Could you check a few things on this model? Use its own coordinates, in mm. Round coordinates to 2 decimals unless told otherwise and drop trailing zeros. Loops run counter-clockwise (first coordinate to the right, second up) from the corner with the lowest first, then second, coordinate; pieces in that order, holes last.
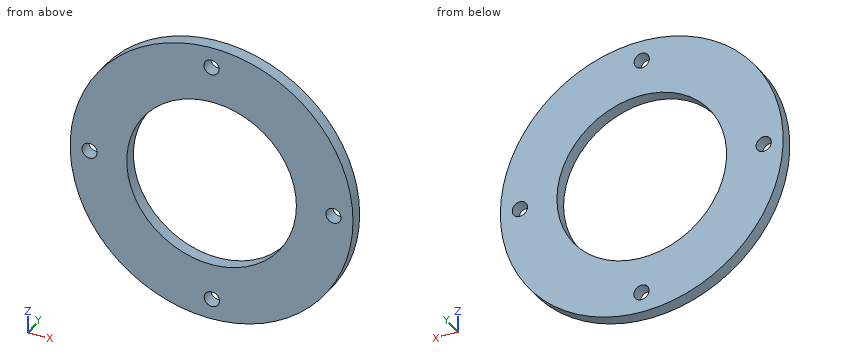
from build123d import *

# Parameters (mm, degrees)
SKETCH1_R                = 32.5
SKETCH1_R_2              = 19.5
BOSS_EXTRUDE2_DEPTH      = 3
SKETCH2_R                = 1.75
CUT_EXTRUDE2_DEPTH       = 1
CUT_EXTRUDE2_DEPTH_BACK  = 4
SKETCH5_R                = 1.75
CUT_EXTRUDE4_DEPTH       = 1
CUT_EXTRUDE4_DEPTH_BACK  = 4
SKETCH13_R               = 1.75
CUT_EXTRUDE12_DEPTH      = 1
CUT_EXTRUDE12_DEPTH_BACK = 4


with BuildPart() as part:
    # Sketch1 → Boss-Extrude2 (new body)
    with BuildSketch(Plane(origin=(0, 0, 0), x_dir=(1, 0, 0), z_dir=(0, 1, 0))):
        Circle(SKETCH1_R)
        Circle(SKETCH1_R_2, mode=Mode.SUBTRACT)
    extrude(amount=BOSS_EXTRUDE2_DEPTH)

    # Sketch2 → Cut-Extrude2 (cut, two sides)
    with BuildSketch(Plane(origin=(0, 3, 0), x_dir=(1, 0, 0), z_dir=(0, 1, 0))) as cut_extrude2_sk:
        with Locations((0, -27.788884535)):
            Circle(SKETCH2_R)
    extrude(amount=CUT_EXTRUDE2_DEPTH, mode=Mode.SUBTRACT)
    extrude(cut_extrude2_sk.sketch, amount=-CUT_EXTRUDE2_DEPTH_BACK, mode=Mode.SUBTRACT)

    # Sketch5 → Cut-Extrude4 (cut, two sides)
    with BuildSketch(Plane(origin=(0, 3, 0), x_dir=(1, 0, 0), z_dir=(0, 1, 0))) as cut_extrude4_sk:
        with Locations((0.057759675, 27.766269398)):
            Circle(SKETCH5_R)
    extrude(amount=CUT_EXTRUDE4_DEPTH, mode=Mode.SUBTRACT)
    extrude(cut_extrude4_sk.sketch, amount=-CUT_EXTRUDE4_DEPTH_BACK, mode=Mode.SUBTRACT)

    # Sketch13 → Cut-Extrude12 (cut, two sides)
    with BuildSketch(Plane(origin=(0, 3, 0), x_dir=(1, 0, 0), z_dir=(0, 1, 0))) as cut_extrude12_sk:
        with Locations((-28.027387252, -0.003979104)):
            Circle(SKETCH13_R)
        with Locations((28.01619309, 0)):
            Circle(SKETCH13_R)
    extrude(amount=CUT_EXTRUDE12_DEPTH, mode=Mode.SUBTRACT)
    extrude(cut_extrude12_sk.sketch, amount=-CUT_EXTRUDE12_DEPTH_BACK, mode=Mode.SUBTRACT)


solid = part.part
Item 1: Will these pins go through, and if not, where does the flat tip stop? pin 1 (12 mm diameter, centred on x = 1, z = 25, fed in from -Y); pin 2 (1.5 mm diameter, centred on y = 1, z = -19.5, fed in from -X); pin 3 (1 mm diameter, centred on x = -11.5, y = 1, fed in from -Z); pin 4 (1 mm diameter, centred on x = 7, y = 1, fed in from -Z).
Results list:
pin 1: stops at y = 0
pin 2: stops at x = -26.55
pin 3: stops at z = -30.58
pin 4: stops at z = -31.84
Item 2: If we section it at A-A, the plane x = -2.5: Please give me the cut outline in (y, z).
Results list:
outline: (0, -32.4) - (3, -32.4) - (3, -19.34) - (0, -19.34) - close; (0, 19.34) - (3, 19.34) - (3, 32.4) - (0, 32.4) - close
Item 3: If we section it at D-D, the plane z = -21.5: Please give me the cut outline in (x, y), then the cut area to 3 significant figures.
Results list:
outline: (-24.37, 0) - (24.37, 0) - (24.37, 3) - (-24.37, 3) - close
area: 146 mm2
Item 4: If I drill on line 1 along Z through (x, y) = (0, 0.6); line 2 along X through (y, z) = (1.45, 0); line 3 along Z through (x, y) = (0.5, 0.75), over which ranges is the centre line in solid material (lowest first)?
Results list:
line 1: z = -32.5 to -29.52, -26.02 to -19.5, 19.5 to 26.04, 29.54 to 32.5
line 2: x = -32.5 to -29.78, -26.28 to -19.5, 19.5 to 26.27, 29.77 to 32.5
line 3: z = -32.5 to -29.46, -26.07 to -19.49, 19.49 to 26.11, 29.47 to 32.5
Item 5: If we section it at B-B, the plane z = -5.5: Please give me the cut outline in (x, y), then the cut area to 3 significant figures.
Results list:
outline: (-32.03, 0) - (-18.71, 0) - (-18.71, 3) - (-32.03, 3) - close; (18.71, 0) - (32.03, 0) - (32.03, 3) - (18.71, 3) - close
area: 79.9 mm2
Item 6: If we section it at C-C, the plane y = 1.7: Please give me the cut outline in (x, z).
Results list:
outline: circle Ø65 at (0, 0); hole circle Ø3.5 at (-28.03, 0); hole circle Ø39 at (0, 0); hole circle Ø3.5 at (0, 27.79); hole circle Ø3.5 at (0.06, -27.77); hole circle Ø3.5 at (28.02, 0)
